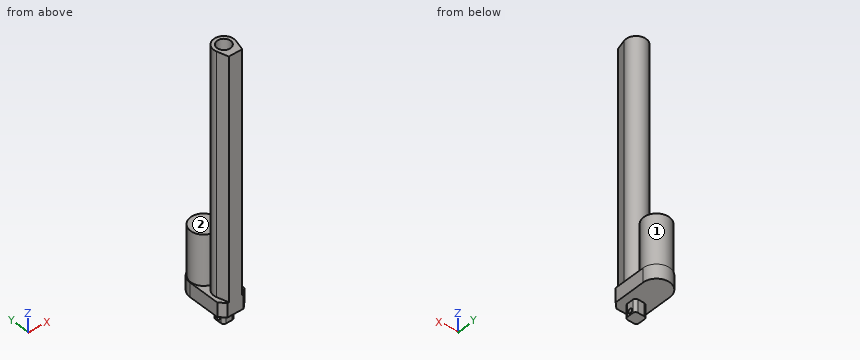
```python
from build123d import *

# Parameters (mm, degrees)
BOSS_EXTRUDE1_DEPTH     = 21
SKETCH2_R               = 19
BOSS_EXTRUDE2_DEPTH     = 74
BOSS_EXTRUDE3_DEPTH     = 355
SKETCH4_W               = 17.3
SKETCH4_H               = 17.3
BOSS_EXTRUDE4_DEPTH     = 19.2
FILLET1_R               = 4
SKETCH5_R               = 10.1
CUT_EXTRUDE1_DEPTH      = 300
SKETCH6_R               = 3.175
CUT_EXTRUDE2_DEPTH      = 21
CUT_EXTRUDE2_DEPTH_BACK = 21


with BuildPart() as part:
    # Sketch1 → Boss-Extrude1 (new body)
    with BuildSketch(Plane.XY):
        with BuildLine():
            Line((-12, -37.5), (12, -37.5))
            Line((12, -37.5), (20, -29.5))
            Line((20, -29.5), (20, 17.5))
            ThreePointArc((20, 17.5), (0, 37.5), (-20, 17.5))
            Line((-20, 17.5), (-20, -29.5))
            Line((-20, -29.5), (-12, -37.5))
        make_face()
    extrude(amount=BOSS_EXTRUDE1_DEPTH)

    # Sketch2 → Boss-Extrude2 (add)
    with BuildSketch(Plane.XY.offset(21)):
        with Locations((0, 17.5)):
            Circle(SKETCH2_R)
    extrude(amount=BOSS_EXTRUDE2_DEPTH)

    # Sketch3 → Boss-Extrude3 (add)
    with BuildSketch(Plane.XY.offset(21)):
        with BuildLine():
            Line((14.449874371, -21.525062814), (10, -37.5))
            Line((10, -37.5), (-10, -37.5))
            Line((-10, -37.5), (-14.449874371, -21.525062814))
            ThreePointArc((-14.449874371, -21.525062814), (0, -2.5), (14.449874371, -21.525062814))
        make_face()
    extrude(amount=BOSS_EXTRUDE3_DEPTH)

    # Sketch4 → Boss-Extrude4 (add)
    with BuildSketch(Plane(origin=(0, 0, 0), x_dir=(-1, 0, 0), z_dir=(0, 0, -1))):
        with Locations((0, -17.85)):
            Rectangle(SKETCH4_W, SKETCH4_H)
    extrude(amount=BOSS_EXTRUDE4_DEPTH)

    # Fillet1
    fillet1_edges = [part.edges().sort_by_distance(p)[0] for p in [
        (-8.65, -26.5, -9.6),
        (-8.65, -9.2, -9.6),
        (8.65, -9.2, -9.6),
        (8.65, -26.5, -9.6),
    ]]
    fillet(fillet1_edges, radius=FILLET1_R)

    # Sketch5 → Cut-Extrude1 (cut)
    with BuildSketch(Plane.XY.offset(376)):
        with Locations((0, -17.5)):
            Circle(SKETCH5_R)
    extrude(amount=-CUT_EXTRUDE1_DEPTH, mode=Mode.SUBTRACT)

    # Sketch6 → Cut-Extrude2 (cut, two sides)
    with BuildSketch(Plane(origin=(0, 0, 0), x_dir=(0, 0, -1), z_dir=(1, 0, 0))) as cut_extrude2_sk:
        with Locations((13.45, -17.85)):
            Circle(SKETCH6_R)
    extrude(amount=CUT_EXTRUDE2_DEPTH, mode=Mode.SUBTRACT)
    extrude(cut_extrude2_sk.sketch, amount=-CUT_EXTRUDE2_DEPTH_BACK, mode=Mode.SUBTRACT)


solid = part.part
```
Build history of the part. All positions in model axes, mm. Face numbers are marked on the shaded views. Round coordinates to 2 decimals unless told otherwise and drop trailing zeros. Loops run counter-clockwise (first coordinate to the right, second up) from the corner with the lowest first, then second, coordinate; pieces in that order, holes last.
Item 1: Drill centre lines: line 1 along Y through (x, z) = (3.75, -13.45) (3 decimals); line 2 along Z through (x, y) = (2.75, -17.85) (3 decimals); line 3 along Y through (x, z) = (0, 313.5). Where is each one in solid material? Low to high.
Item 2: Saw through at A-A (z = 133). List the corners of the cut face in (x, y).
Item 3: Pin check, flat tips, straight feed: P1, Ø6, axis at y = -27.5, z = 25.5, coming from the +X side; P2, Ø3, axis at x = -1, z = -5, coming from the +Y side; P3, Ø16, axis at x = 0, y = -17.5, coming from the +Z side; P4, Ø5, axis at y = -17.85, z = -13.45, coming from the +X side. Stop position of each tip, or through.
Item 4: Two-plate mould, pull along Y, no slides. Class the marked faces 1 and 2: released by +Y, released by -Y, zero draft, split by the parting line, or undercut.
Item 5: Saw through at B-B (y = 13). List the corners of the cut face in (x, z), then the cut area to 3 significant figures.
Worked answers:
1. line 1: y = -26.5 to -21.025, -14.675 to -9.2
1. line 2: z = -19.2 to -16.625, -10.275 to 76
1. line 3: y = -37.5 to -27.6, -7.4 to -2.5
2. outline: (-14.45, -21.53) - (-10, -37.5) - (10, -37.5) - (14.45, -21.53) arc R15 ccw (long way) to start; hole circle Ø20.2 at (0, -17.5)
3. P1: stops at x = 13.62
3. P2: stops at y = -9.2
3. P3: stops at z = 76
3. P4: passes through
4. face 1: undercut
4. face 2: zero draft
5. outline: (-20, 0) - (20, 0) - (20, 21) - (18.46, 21) - (18.46, 95) - (-18.46, 95) - (-18.46, 21) - (-20, 21) - close
5. area: 3,570 mm2
